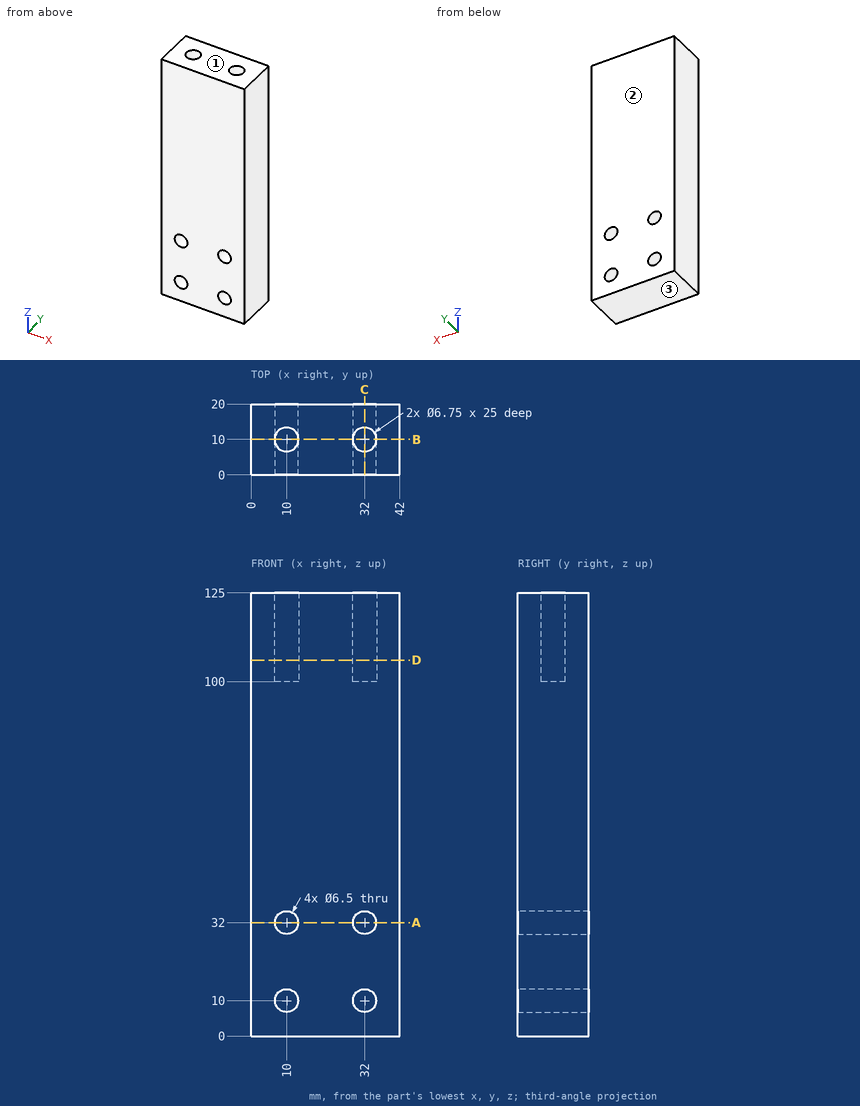
Can you work these out from the drawing? Everything is in mm from the part's minimum corner. Round coordinates to 2 decimals unless told otherwise and drop trailing zeros. Order: outer loops, then holes, each group sorted by start corner. A loop starts at its lowest first (then second) coordinate and runs counter-clockwise, first axis right, second up. Notation, with made-up numbers: (-1, -39) -> (30, -39) arc R10 cw to (30, -20) -> close; hole circle Ø10 at (-39.75, -19). An arc over 180 degrees is marked (long way). Return JSON: item names as keys, results as strings. Group by question number.
1. I need wall thicknesses on line 1 (X direction, y = 18, z = 32); line 2 (Y direction, x = 10, z = 114) (3 decimals); line 3 (Z direction, x = 29, y = 15.5). Which ranges of each line are inside material? Lowest first, please. Write a range as [from, to].
2. If we section it at A-A, the plane z = 32: Write out the boundary of the cut face in (x, y), then the cut area to 3 significant figures.
3. Will these pins go through, and if not, where does the flat tip stop? pin 1 (1 mm diameter, centred on x = 9, z = 100.5, fed in from -Y); pin 2 (5.5 mm diameter, centred on x = 10, y = 10, fed in from +Z); pin 3 (6 mm diameter, centred on x = 32, z = 32, fed in from -Y).
4. If we section it at D-D, the plane z = 106: Write out the boundary of the cut face in (x, y) (3 decimals).
5. We'd pull the mould along Z, two halves only. Please class the marked faces 1, 2 and 3: released by +Z, released by -Z, zero draft, split by the parting line, or undercut.
6. If we section it at B-B, the plane y = 10: Write out the boundary of the cut face in (x, z) (3 decimals), then the cut area to 3 significant figures.
7. If we section it at C-C, the plane x = 32: Write out the boundary of the cut face in (y, z) (3 decimals), then the cut area to 3 significant figures.
Output values:
{
 "1": {"line 1": "[0, 6.75], [13.25, 28.75], [35.25, 42]", "line 2": "[0, 6.625], [13.375, 20]", "line 3": "[0, 8.75], [11.25, 30.75], [33.25, 125]"},
 "2": {"outline": "(0, 0) -> (6.75, 0) -> (6.75, 20) -> (0, 20) -> close; (13.25, 0) -> (28.75, 0) -> (28.75, 20) -> (13.25, 20) -> close; (35.25, 0) -> (42, 0) -> (42, 20) -> (35.25, 20) -> close", "area": "580 mm²"},
 "3": {"pin 1": "y = 0", "pin 2": "z = 100", "pin 3": "through"},
 "4": {"outline": "(0, 0) -> (42, 0) -> (42, 20) -> (0, 20) -> close; hole circle Ø6.75 at (10, 10); hole circle Ø6.75 at (32, 10)"},
 "5": {"face 1": "released by +Z", "face 2": "zero draft", "face 3": "released by -Z"},
 "6": {"outline": "(0, 0) -> (42, 0) -> (42, 125) -> (35.375, 125) -> (35.375, 100) -> (28.625, 100) -> (28.625, 125) -> (13.375, 125) -> (13.375, 100) -> (6.625, 100) -> (6.625, 125) -> (0, 125) -> close; hole circle Ø6.5 at (10, 10); hole circle Ø6.5 at (10, 32); hole circle Ø6.5 at (32, 10); hole circle Ø6.5 at (32, 32)", "area": "4,780 mm²"},
 "7": {"outline": "(0, 0) -> (20, 0) -> (20, 6.75) -> (0, 6.75) -> close; (0, 13.25) -> (20, 13.25) -> (20, 28.75) -> (0, 28.75) -> close; (0, 35.25) -> (20, 35.25) -> (20, 125) -> (13.375, 125) -> (13.375, 100) -> (6.625, 100) -> (6.625, 125) -> (0, 125) -> close", "area": "2,070 mm²"}
}
